Read the model definition and answer for the solid it produces. Units are mm, in the model's axes. Face numbers are marked on the shaded views. A direction names the side the tool comes from. Round coordinates to 2 decimals unless told otherwise and drop trailing zeros. One line per item, written item: value. Start each with the question number.
(1) Find the intervals of material crossed by L1, parallel to Y at x = -8, z = 3.2; L2, parallel to X at y = -1.5, z = 1.85; L3, parallel to X at y = -1.25, z = 1.75, in increasing order.
(2) Flat-ended cylindrical pins translate along their axes: pin 1 Ø1.2 at (x, y) = (24.05, -16.79) entering from -Z; pin 2 Ø0.9 at (x, z) = (-22.5, 4) entering from +Y; pin 3 Ø1.5 at (x, z) = (-12.5, 3.5) entering from -Y. Find the tip coordinate at first contact, or state that the pin passes through.
(3) The mould has two halves that part along X. Classify the marked faces 4, 5, 6 and 7: +X half, -X half, draft (parallel to the pull), parting line (faces both ways), or undercut.
(4) For the marked faces 1, 2 and 3, determine the directions among +Z, -Z, +X, -X, +Y, -Y from which every point of the face is accessible in a straight line to the end or side of a thin tool.
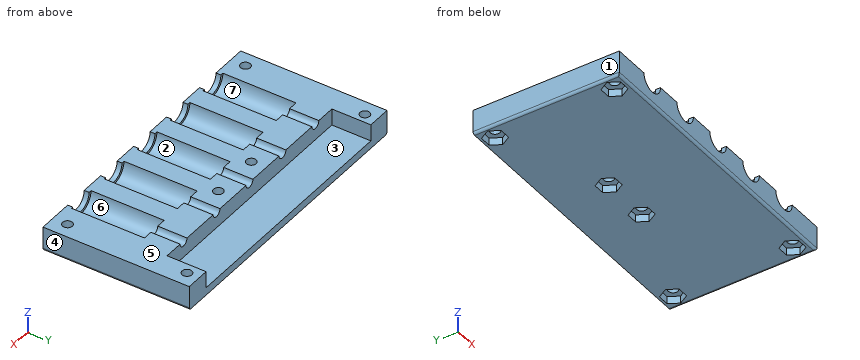
from build123d import *

# Parameters (mm, degrees)
F0_W      = 60
F0_H      = 25
F1_DEPTH  = 5
F2_R      = 2.5
F3_DEPTH  = 10
F5_R      = 3
F6_DEPTH  = 15
F7_R      = 1.05
F8_DEPTH  = 29
F9_W      = 50
F9_H      = 3.4154356362
F10_DEPTH = 3
F11_DEPTH = 5
F12_R     = 0.5
F14_R     = 1
F13_R     = 1
F15_DEPTH = 5.001
F16_R     = 1
F17_DEPTH = 5
F19_DEPTH = 1.5


with BuildPart() as f1:
    # F0 (on Top) → F1 (new body)
    with BuildSketch(Plane.XY):
        with Locations((-2.9453901201, -7.2920476746)):
            Rectangle(F0_W, F0_H)
    extrude(amount=F1_DEPTH)

    # F2 (on face) → F3 (cut)
    with BuildSketch(Plane.XZ.offset(19.7920476746)):
        with Locations((-22.9453901201, 5)):
            Circle(F2_R)
        with Locations((-12.9453901201, 5)):
            Circle(F2_R)
        with Locations((-2.9453901201, 5)):
            Circle(F2_R)
        with Locations((7.0546098799, 5)):
            Circle(F2_R)
        with Locations((17.0546098799, 5)):
            Circle(F2_R)
    extrude(amount=-F3_DEPTH, mode=Mode.SUBTRACT)

    # F5 (on offset) → F6 (cut)
    with BuildSketch(Plane.XZ.offset(18.7920476746)):
        with Locations((-23.0476632714, 5.0127296709)):
            Circle(F5_R)
        with Locations((-13.0476632714, 5.0127296709)):
            Circle(F5_R)
        with Locations((-3.0476632714, 5.0127296709)):
            Circle(F5_R)
        with Locations((6.9523367286, 5.0127296709)):
            Circle(F5_R)
        with Locations((16.9523367286, 5.0127296709)):
            Circle(F5_R)
    extrude(amount=-F6_DEPTH, mode=Mode.SUBTRACT)

    # F7 (on face) → F8 (cut)
    with BuildSketch(Plane.XZ.offset(3.7920476746)):
        with Locations((-23.0476632714, 5.0127296709)):
            Circle(F7_R)
        with Locations((-13.0476632714, 5.0127296709)):
            Circle(F7_R)
        with Locations((-3.0476632714, 5.0127296709)):
            Circle(F7_R)
        with Locations((6.9523367286, 5.0127296709)):
            Circle(F7_R)
        with Locations((16.9523367286, 5.0127296709)):
            Circle(F7_R)
    extrude(amount=-F8_DEPTH, mode=Mode.SUBTRACT)

    # F9 (on face) → F10 (cut)
    with BuildSketch(Plane(origin=(0, 5.2079523254, 0), x_dir=(-1, 0, 0), z_dir=(0, 1, 0))):
        with Locations((3.0476632714, 3.2922821819)):
            Rectangle(F9_W, F9_H)
    extrude(amount=-F10_DEPTH, mode=Mode.SUBTRACT)

    # F11 (add): a face of the model
    f11_faces = [f1.faces().sort_by_distance(p)[0] for p in [
        (-2.8102387692, 5.2079523254, 1.4530193808),
    ]]
    extrude(f11_faces, amount=F11_DEPTH)

    # F12
    f12_edges = [f1.edges().sort_by_distance(p)[0] for p in [
        (27.05461, -4.792048, 0),
        (-2.94539, -19.792048, 0),
        (-32.94539, -4.792048, 0),
    ]]
    fillet(f12_edges, radius=F12_R)

    # F14 (on face) + F13 (on face) → F15 (cut, through all)
    with BuildSketch(Plane(origin=(0, 0, 0), x_dir=(1, 0, 0), z_dir=(0, 0, -1))):
        with Locations((-29.9453901201, -7.7079523254)):
            Circle(F14_R)
        with Locations((24.0546098799, -7.7079523254)):
            Circle(F14_R)
    with BuildSketch(Plane(origin=(0, 0, 0), x_dir=(1, 0, 0), z_dir=(0, 0, -1))):
        with Locations((-29.9453901201, 16.7920476746)):
            Circle(F13_R)
        with Locations((24.0546098799, 16.7920476746)):
            Circle(F13_R)
    extrude(amount=-F15_DEPTH, mode=Mode.SUBTRACT)

    # F16 (on face) → F17 (cut)
    with BuildSketch(Plane.XY.offset(5)):
        with Locations((1.9524138955, -0.7920476746)):
            Circle(F16_R)
        with Locations((-8.0475861045, -0.7920476746)):
            Circle(F16_R)
    extrude(amount=-F17_DEPTH, mode=Mode.SUBTRACT)

    # F18 (on face) → F19 (cut)
    with BuildSketch(Plane(origin=(0, 0, 0), x_dir=(1, 0, 0), z_dir=(0, 0, -1))):
        Polygon((25.2093104182, -5.7079523254), (22.8999093415, -5.7079523254), (21.7452088031, -7.7079523254), (22.8999093415, -9.7079523254), (25.2093104182, -9.7079523254), (26.3640109566, -7.7079523254), align=None)
        Polygon((25.2093104182, 18.7920476746), (22.8999093415, 18.7920476746), (21.7452088031, 16.7920476746), (22.8999093415, 14.7920476746), (25.2093104182, 14.7920476746), (26.3640109566, 16.7920476746), align=None)
        Polygon((-28.7906895818, 18.7920476746), (-31.1000906585, 18.7920476746), (-32.2547911969, 16.7920476746), (-31.1000906585, 14.7920476746), (-28.7906895818, 14.7920476746), (-27.6359890434, 16.7920476746), align=None)
        Polygon((-31.1000906585, -9.7079523254), (-28.7906895818, -9.7079523254), (-27.6359890434, -7.7079523254), (-28.7906895818, -5.7079523254), (-31.1000906585, -5.7079523254), (-32.2547911969, -7.7079523254), align=None)
        Polygon((0.7977133571, -1.2079523254), (3.1071144338, -1.2079523254), (4.2618149722, 0.7920476746), (3.1071144338, 2.7920476746), (0.7977133571, 2.7920476746), (-0.3569871813, 0.7920476746), align=None)
        Polygon((-9.2022866429, -1.2079523254), (-6.8928855662, -1.2079523254), (-5.7381850278, 0.7920476746), (-6.8928855662, 2.7920476746), (-9.2022866429, 2.7920476746), (-10.3569871813, 0.7920476746), align=None)
    extrude(amount=-F19_DEPTH, mode=Mode.SUBTRACT)


solid = f1.part
Here are the results:
1. L1: -19.79 to -1.79, 0.21 to 2.21
1. L2: -32.95 to -8.75, -7.34 to 1.25, 2.66 to 27.05
1. L3: -32.95 to -8.94, -7.16 to 1.06, 2.84 to 27.05
2. pin 1: through
2. pin 2: y = 2.21
2. pin 3: y = -3.79
3. face 4: +X half
3. face 5: draft
3. face 6: undercut
3. face 7: undercut
4. face 1: +Z, -Z, -X, +Y, -Y
4. face 2: +Z
4. face 3: +Z, +Y
